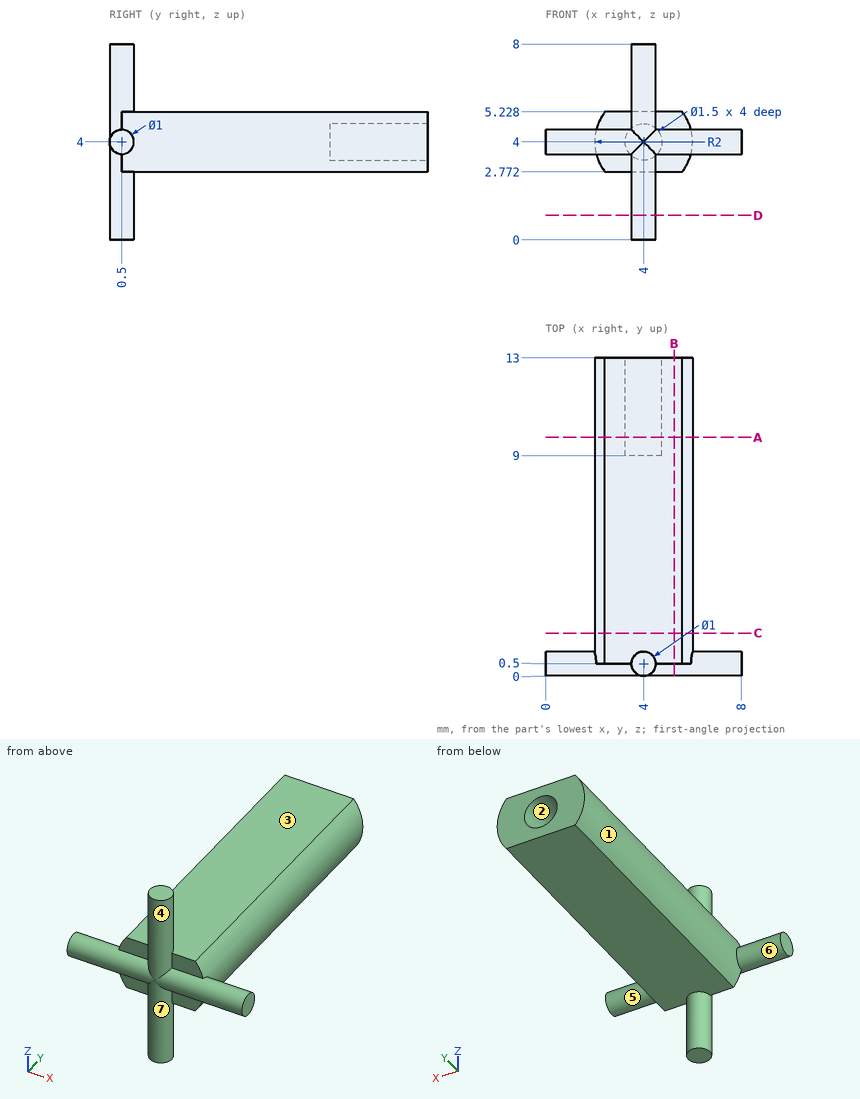
Part print with two shaded views. Sizes in mm from the minimum x, y, z corner. A direction names the side the tool comes from. Round coordinates to 2 decimals unless told otherwise and drop trailing zeros. Loops run counter-clockwise (first coordinate to the right, second up) from the corner with the lowest first, then second, coordinate; pieces in that order, holes last. Notation, with made-up numbers: (-40, 51) - (-18, 51) arc R11 cw to (-18, 70) - close; hole circle Ø8 at (24.5, -28). An arc over 180 degrees is marked (long way). Put each result on its own line as item: value.
1. Two-plate mould, pull along X, no slides. Class the marked faces 1, 2 and 3: released by +X, released by -X, zero draft, split by the parting line, or undercut.
Geometry check:
face 1: released by -X
face 2: undercut
face 3: zero draft
2. Slice it at A-A on y = 9.75. List the corners of the cut face in (x, z).
Geometry check:
outline: (2.42, 2.77) - (5.58, 2.77) arc R2 ccw to (5.58, 5.23) - (2.42, 5.23) arc R2 ccw to start; hole circle Ø1.5 at (4, 4)
3. Wall check: line 1 (X direction, y = 11.75, z = 4); line 2 (Z direction, x = 3.25, y = 1.5); line 3 (Y direction, x = 5, z = 3.25). Give the ranges that are in metal, low to high.
Geometry check:
line 1: 2 to 3.25, 4.75 to 6
line 2: 2.77 to 5.23
line 3: 0.5 to 13
4. Pin check, flat tips, straight feed: P1, Ø2.5, axis at x = 3.5, y = 8, coming from the +Z side; P2, Ø4, axis at y = 6, z = 3, coming from the -X side; P3, Ø3.5, axis at x = 4, y = 7.5, coming from the -Z side. Stop position of each tip, or through.
Geometry check:
P1: z = 5.23
P2: x = 2
P3: z = 2.77
5. Slice it at C-C on y = 1.75. List the corners of the cut face in (x, z).
Geometry check:
outline: (2.42, 2.77) - (5.58, 2.77) arc R2 ccw to (5.58, 5.23) - (2.42, 5.23) arc R2 ccw to start
6. Slice it at D-D on z = 1. List the corners of the cut face in (x, y).
Geometry check:
outline: circle Ø1 at (4, 0.5)
7. 3-axis set-ups, long thin cutter, end or side, ignore diameter. For the marked faces 4, 5, 6 and 7: which of +Z, -Z, +X, -X, +Y, -Y reach the whole face in a straight line?
Geometry check:
face 4: +Z
face 5: +X
face 6: -X
face 7: -Z
8. Slice it at B-B on x = 5.25. List the corners of the cut face in (y, z).
Geometry check:
outline: (0.5, 2.77) - (13, 2.77) - (13, 5.23) - (0.5, 5.23) - (0.5, 4.5) arc R0.5 ccw to (0.5, 3.5) - close
